The model under review builds one solid part; all positions refer to its coordinate system, in mm. A direction names the side the tool comes from. Coordinates: 2 decimals unless noted, no trailing zeros. Write each loop counter-clockwise with the first axis right and the second up, starting at its lowest first coordinate (ties: lowest second). Pieces come first, ordered by that corner, then holes.
1) Mouldability with a two-part tool opening along Z and no side actions: class faces 4 (the flat face through (0, 13, 0)), 5 (the flat face through (21, 25, 29)), 6 (the cylindrical face through (-15.93, 35.88, 11.92)), 7 (the cylindrical face through (-15.912, 37.92, 40.794)) as released by +Z, released by -Z, zero draft, split by the parting line, or undercut.
2) Add section B-B, the plane z = 32.5. State the section outline as (x, y) points (3 decimals), then the cut area to 3 significant figures.
3) For line 1 (Z direction, x = -3.5, y = -13); line 2 (Z direction, x = -0.5, y = -15.5); line 3 (X direction, y = 34, z = 39) (3 decimals), list the stretches that pass through material, from the lowest coordinate up.
4) Machinability: for faces 1 (the flat face through (-10.635, -13, 29)), 2 (the flat face through (0, -26, 29)), 3 (the flat face through (10.635, -13, 29)), which of the approach directions +Z, -Z, +X, -X, +Y, -Y give a long, thin tool a straight path to every point of the face, cutting with its end or side? Answer none if there is none.
5) Add section D-D, the plane y = 44. State the section outline as (x, z) points (3 decimals), then the cut area to 3 significant figures.
6) Add section C-C, the plane x = 4.5. State the section outline as (y, z) points.
7) For P1, Ø3, axis at x = -16, z = 39, coming from the -Y side; P2, Ø4, axis at y = -14, z = 47.5, coming from the -X side (3 decimals); P3, Ø8, axis at y = -13, z = 14.4, coming from the +X side (3 decimals); P4, Ø3.5, axis at y = -13, z = 43.9, coming from the +X side, all flat-tipped, find the tip position at first contact; note any pin that passes through.
8) Add section A-A, the plane y = -13. State the section outline as (x, z) points (3 decimals).
from build123d import *

# Parameters (mm, degrees)
F1_DEPTH = 58.3
F2_R     = 3
F3_DEPTH = 25
F4_R     = 3
F5_DEPTH = 25
F6_DEPTH = 100


with BuildPart() as f1:
    # F0 (on Top) → F1 (new body)
    with BuildSketch(Plane.XY):
        Polygon((-10.635, 0), (-10.635, -26), (10.635, -26), (10.635, 0), (21, 0), (21, 50), (11.135, 50), (10.875, 24), (0, 24.10875), (-10.875, 24), (-11.135, 50), (-21, 50), (-21, 0), align=None)
    extrude(amount=F1_DEPTH)

    # F2 (on face) → F3 (cut)
    with BuildSketch(Plane(origin=(-10.635, 0, 0), x_dir=(0, -1, 0), z_dir=(-1, 0, 0))):
        with Locations((13, 14.4)):
            Circle(F2_R)
        with Locations((13, 43.9)):
            Circle(F2_R)
    extrude(amount=-F3_DEPTH, mode=Mode.SUBTRACT)

    # F4 (on face) → F5 (cut)
    with BuildSketch(Plane(origin=(10.633937, -0.106339, 0), x_dir=(-0.01, -0.99995, 0), z_dir=(-0.99995, 0.01, 0))):
        with Locations((-37.108195, 14.577401)):
            Circle(F4_R)
        with Locations((-37.108195, 43.722599)):
            Circle(F4_R)
    extrude(amount=-F5_DEPTH, mode=Mode.SUBTRACT)

    # F4 (on face) → F6 (cut)
    with BuildSketch(Plane(origin=(10.633937, -0.106339, 0), x_dir=(-0.01, -0.99995, 0), z_dir=(-0.99995, 0.01, 0))):
        with Locations((-37.108195, 43.722599)):
            Circle(F4_R)
        with Locations((-37.108195, 14.577401)):
            Circle(F4_R)
    extrude(amount=F6_DEPTH, mode=Mode.SUBTRACT)


solid = f1.part
Geometry results:
1. face 4: released by -Z
1. face 5: zero draft
1. face 6: undercut
1. face 7: undercut
2. outline: (-21, 0) - (-10.635, 0) - (-10.635, -26) - (10.635, -26) - (10.635, 0) - (21, 0) - (21, 50) - (11.135, 50) - (10.875, 24) - (0, 24.109) - (-10.875, 24) - (-11.135, 50) - (-21, 50) - close
2. area: 2,080 mm2
3. line 1: z = 0 to 11.4, 17.4 to 40.9, 46.9 to 58.3
3. line 2: z = 0 to 12.74, 16.06 to 42.24, 45.56 to 58.3
3. line 3: x = -21 to -10.975, 10.975 to 21
4. face 1: +Z, -Z, -X, -Y
4. face 2: +Z, -Z, +X, -X, -Y
4. face 3: +Z, -Z, +X, -Y
5. outline: (-21, 0) - (-11.075, 0) - (-11.075, 58.3) - (-21, 58.3) - close; (11.075, 0) - (21, 0) - (21, 58.3) - (11.075, 58.3) - close
5. area: 1,160 mm2
6. outline: (-26, 0) - (24.06, 0) - (24.06, 58.3) - (-26, 58.3) - close; hole circle Ø6 at (-13, 14.4); hole circle Ø6 at (-13, 43.9)
7. P1: stops at y = 0
7. P2: stops at x = -10.635
7. P3: stops at x = 10.635
7. P4: passes through
8. outline: (-10.635, 0) - (10.635, 0) - (10.635, 11.4) - (-10.635, 11.4) - close; (-10.635, 17.4) - (10.635, 17.4) - (10.635, 40.9) - (-10.635, 40.9) - close; (-10.635, 46.9) - (10.635, 46.9) - (10.635, 58.3) - (-10.635, 58.3) - close
